```python
from build123d import *

# Parameters (mm, degrees)
F1_DEPTH = 0.5
F2_W     = 15
F2_H     = 0.5
F3_DEPTH = 4
F4_R     = 2.6209807332
F5_DEPTH = 25
F6_R     = 1.7070089516
F7_DEPTH = 25


with BuildPart() as f1:
    # F0 (on Right) → F1 (new body, symmetric)
    with BuildSketch(Plane.YZ):
        Polygon((-15, 0), (0, 0), (3.2893587091, 19.7276485999), (-0.7106412909, 19.7276485999), (-15, 3), align=None)
    extrude(amount=F1_DEPTH, both=True)

    # F2 (on Right) → F3 (join, symmetric)
    with BuildSketch(Plane.YZ):
        with Locations((-7.5, -0.25)):
            Rectangle(F2_W, F2_H)
    extrude(amount=F3_DEPTH, both=True)

    # F4 (on face) → F5 (cut)
    with BuildSketch(Plane.YZ.offset(0.5)):
        with BuildLine():
            ThreePointArc((-0.4529937069, 2.964487765), (-3.0851524789, 5.5966465369), (-5.7173112508, 2.964487765))
            ThreePointArc((-5.7173112508, 2.964487765), (-3.0851524789, 0.332328993), (-0.4529937069, 2.964487765))
        make_face()
        with Locations((-11.2699056044, 2.964487765)):
            Circle(F4_R)
        with BuildLine():
            Line((-3.3178431468, 10.4724832487), (-5.453436658, 6.3182523414))
            ThreePointArc((-5.453436658, 6.3182523414), (-3.16893319, 6.4018223867), (-2.0501317095, 8.395367795))
            ThreePointArc((-2.0501317095, 8.395367795), (-2.392094494, 9.6120745074), (-3.3178431468, 10.4724832487))
        make_face()
        with BuildLine():
            ThreePointArc((-3.3178431468, 10.4724832487), (-6.462755356, 9.4631645506), (-5.453436658, 6.3182523414))
            Line((-5.453436658, 6.3182523414), (-3.3178431468, 10.4724832487))
        make_face()
        with BuildLine():
            Line((-0.6935525003, 15.577344851), (-2.6388447391, 11.7932946093))
            ThreePointArc((-2.6388447391, 11.7932946093), (-0.5579118075, 11.8694177852), (0.4611940407, 13.6853197301))
            ThreePointArc((0.4611940407, 13.6853197301), (0.1497033252, 14.7936065423), (-0.6935525003, 15.577344851))
        make_face()
        with BuildLine():
            ThreePointArc((-0.6935525003, 15.577344851), (-3.5582237405, 14.6579658495), (-2.6388447391, 11.7932946093))
            Line((-2.6388447391, 11.7932946093), (-0.6935525003, 15.577344851))
        make_face()
        with BuildLine():
            ThreePointArc((1.8837464303, 18.1615501642), (-0.0156576164, 19.2275183887), (0.0639659937, 17.0508962192))
            ThreePointArc((0.0639659937, 17.0508962192), (1.285512338, 17.0955819397), (1.8837464303, 18.1615501642))
        make_face()
    extrude(amount=-F5_DEPTH, mode=Mode.SUBTRACT)

    # F6 (on face) → F7 (cut)
    with BuildSketch(Plane.YZ.offset(0.5)):
        with Locations((-8.3660604432, 6.5863626078)):
            Circle(F6_R)
    extrude(amount=-F7_DEPTH, mode=Mode.SUBTRACT)


solid = f1.part
```
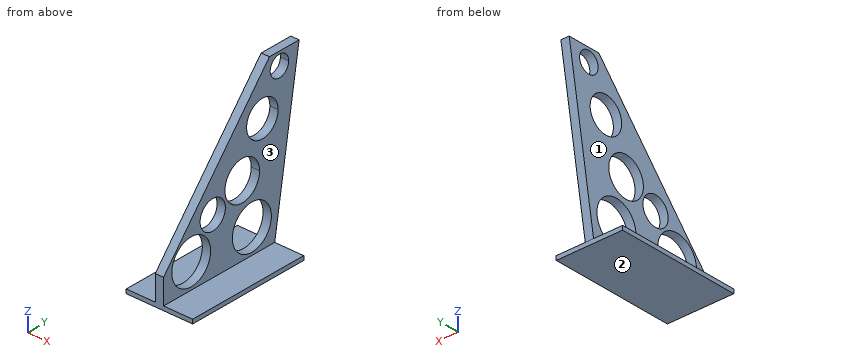
The model under review builds one solid part; all positions refer to its coordinate system, in mm. Face numbers are marked on the shaded views. A direction names the side the tool comes from. Round coordinates to 2 decimals unless told otherwise and drop trailing zeros. Write each loop counter-clockwise with the first axis right and the second up, starting at its lowest first coordinate (ties: lowest second). Pieces come first, ordered by that corner, then holes.
(1) We need section D-D on y = -12. Give the boundary of the cut face in (x, z).
(2) We need section A-A on y = -9.5. Give the boundary of the cut face in (x, z), and give its area (3 significant figures).
(3) Wall thickness on L1, parallel to Z at x = -1.25, y = -6.25; L2, parallel to X at y = 0, z = 1.25; L3, parallel to Z at x = -0.25, y = -6.25: over which ranges is each line inside the solid? List them lowest first.
(4) Machinability: for the marked faces 1, 2 and 3, which of the approach directions +Z, -Z, +X, -X, +Y, -Y give a long, thin tool a straight path to every point of the face, cutting with its end or side? Answer none if there is none.
(5) We need section C-C on z = 2. Give the boundary of the cut face in (x, y).
(6) Insertion check: pin 1 (3 mm diameter, centred on y = 0.63, z = 18.16, fed in from -X); pin 2 (4 mm diameter, centred on x = 2, y = -9, fed in from +Z); pin 3 (1 mm diameter, centred on x = -2, y = -4.5, fed in from +Z). Each pin has a flat end and moves straight along its axis. Give the tip position at first contact, or say it passes through.
(7) We need section B-B on z = 12.75. Give the boundary of the cut face in (x, y).
Findings below:
1. outline: (-4, -0.5) - (4, -0.5) - (4, 0) - (0.5, 0) - (0.5, 0.45) - (-0.5, 0.45) - (-0.5, 0) - (-4, 0) - close; (-0.5, 5.48) - (0.5, 5.48) - (0.5, 6.51) - (-0.5, 6.51) - close
2. outline: (-4, -0.5) - (4, -0.5) - (4, 0) - (0.5, 0) - (0.5, 1.03) - (-0.5, 1.03) - (-0.5, 0) - (-4, 0) - close; (-0.5, 4.9) - (0.5, 4.9) - (0.5, 5.31) - (-0.5, 5.31) - close; (-0.5, 7.86) - (0.5, 7.86) - (0.5, 9.44) - (-0.5, 9.44) - close
2. area: 7.02 mm2
3. L1: z = -0.5 to 0
3. L2: x = -0.5 to 0.5
3. L3: z = -0.5 to 6.99, 9.8 to 13.24
4. face 1: +Z, -X, +Y, -Y
4. face 2: -Z, +X, -X, +Y, -Y
4. face 3: +Z, +X, +Y, -Y
5. outline: (-0.5, -15) - (0.5, -15) - (0.5, -13.71) - (-0.5, -13.71) - close; (-0.5, -8.83) - (0.5, -8.83) - (0.5, -5.53) - (-0.5, -5.53) - close; (-0.5, -0.64) - (0.5, -0.64) - (0.5, 0.33) - (-0.5, 0.33) - close
6. pin 1: stops at x = -0.5
6. pin 2: stops at z = 11.57
6. pin 3: stops at z = 0
7. outline: (-0.5, -6.67) - (0.5, -6.67) - (0.5, -3.58) - (-0.5, -3.58) - close; (-0.5, 0.24) - (0.5, 0.24) - (0.5, 2.13) - (-0.5, 2.13) - close
